Input: part model. Units: mm. Frame: model coordinates. A direction names the side the tool comes from. Give positions to 0.01 mm unless a question says otherwise; leave off trailing zeros. Write each loop counter-clockwise with the first axis right and the second up, starting at its lowest first coordinate (ties: lowest second). Pieces come first, ordered by that corner, then holes. Notation, with made-up numbers: (-7, 47.25) - (47, 47.25) arc R15 cw to (47, 72.25) - close; hole circle Ø8 at (78.25, 25.25). An arc over 180 degrees is marked (long way). Answer as a JSON object with one key per item and string values. Group by question number.
from build123d import *

# Parameters (mm, degrees)
SKETCH1_W           = 75
SKETCH1_H           = 80
BOSS_EXTRUDE1_DEPTH = 3
SKETCH2_W           = 17
SKETCH2_H           = 80
BOSS_EXTRUDE2_DEPTH = 3
SKETCH7_W           = 25
SKETCH7_H           = 80
SKETCH7_W_2         = 14.8
SKETCH7_H_2         = 17
BOSS_EXTRUDE6_DEPTH = 3
SKETCH8_W           = 21.55
SKETCH8_H           = 23.85
SKETCH8_W_2         = 17.55
SKETCH8_H_2         = 19.85
BOSS_EXTRUDE7_DEPTH = 10
SKETCH9_W           = 12.5
SKETCH9_H           = 2.5
CUT_EXTRUDE3_DEPTH  = 23.85
SKETCH10_W          = 1.375
SKETCH10_H          = 19.85
BOSS_EXTRUDE8_DEPTH = 6.5
SKETCH11_W          = 20
SKETCH11_H          = 80
SKETCH11_R          = 2.7
BOSS_EXTRUDE9_DEPTH = 3
SKETCH3_W           = 8
SKETCH3_H           = 15
BOSS_EXTRUDE3_DEPTH = 3
SKETCH5_W           = 69
SKETCH5_H           = 17
SKETCH5_R           = 2.6
SKETCH5_W_2         = 25
BOSS_EXTRUDE4_DEPTH = 3
SKETCH21_R          = 2.7
CUT_EXTRUDE5_DEPTH  = 3


with BuildPart() as part:
    # Sketch1 → Boss-Extrude1 (new body)
    with BuildSketch(Plane.XY):
        with Locations((0, 40)):
            Rectangle(SKETCH1_W, SKETCH1_H)
        Polygon((4.25, 23.5), (20.75, 23.5), (26.5, 30), (26.5, 72), (-1.5, 72), (-1.5, 30), align=None, mode=Mode.SUBTRACT)
    extrude(amount=BOSS_EXTRUDE1_DEPTH)

    # Sketch2 → Boss-Extrude2 (add)
    with BuildSketch(Plane(origin=(37.5, 0, 0), x_dir=(0, 0, -1), z_dir=(1, 0, 0))):
        with Locations((8.5, 40)):
            Rectangle(SKETCH2_W, SKETCH2_H)
    boss_extrude2 = extrude(amount=-BOSS_EXTRUDE2_DEPTH)

    # Mirror1: Boss-Extrude2 across plane
    add(boss_extrude2.mirror(Plane(origin=(0, 0, 0), x_dir=(0, 0, 1), z_dir=(1, 0, 0))))

    # Sketch7 → Boss-Extrude6 (add)
    with BuildSketch(Plane.XY.offset(3)):
        with Locations((50, 40)):
            Rectangle(SKETCH7_W, SKETCH7_H)
        with Locations((50, 48.001193432)):
            Rectangle(SKETCH7_W_2, SKETCH7_H_2, mode=Mode.SUBTRACT)
    extrude(amount=-BOSS_EXTRUDE6_DEPTH)

    # Sketch8 → Boss-Extrude7 (add)
    with BuildSketch(Plane(origin=(0, 0, 0), x_dir=(-1, 0, 0), z_dir=(0, 0, -1))):
        with Locations((-50, 48.001193432)):
            Rectangle(SKETCH8_W, SKETCH8_H)
        with Locations((-50, 48.001193432)):
            Rectangle(SKETCH8_W_2, SKETCH8_H_2, mode=Mode.SUBTRACT)
    extrude(amount=BOSS_EXTRUDE7_DEPTH)

    # Sketch9 → Cut-Extrude3 (cut)
    with BuildSketch(Plane(origin=(0, 59.926193432, 0), x_dir=(1, 0, 0), z_dir=(0, 1, 0))):
        with Locations((50, 4.75)):
            Rectangle(SKETCH9_W, SKETCH9_H)
    extrude(amount=-CUT_EXTRUDE3_DEPTH, mode=Mode.SUBTRACT)

    # Sketch10 → Boss-Extrude8 (add)
    with BuildSketch(Plane(origin=(0, 0, 0), x_dir=(-1, 0, 0), z_dir=(0, 0, -1))):
        with Locations((-41.9125, 48.001193432)):
            Rectangle(SKETCH10_W, SKETCH10_H)
        with Locations((-58.0875, 48.001193432)):
            Rectangle(SKETCH10_W, SKETCH10_H)
    extrude(amount=BOSS_EXTRUDE8_DEPTH)

    # Sketch11 → Boss-Extrude9 (add)
    with BuildSketch(Plane(origin=(62.5, 0, 0), x_dir=(0, 0, -1), z_dir=(1, 0, 0))):
        with Locations((7, 40)):
            Rectangle(SKETCH11_W, SKETCH11_H)
        with Locations((7, 15)):
            Circle(SKETCH11_R, mode=Mode.SUBTRACT)
        with Locations((7, 65)):
            Circle(SKETCH11_R, mode=Mode.SUBTRACT)
    extrude(amount=BOSS_EXTRUDE9_DEPTH)

    # Sketch3 → Boss-Extrude3 (add)
    with BuildSketch(Plane(origin=(0, 0, 0), x_dir=(-1, 0, 0), z_dir=(0, 0, -1))):
        with Locations((-30.5, 49)):
            Rectangle(SKETCH3_W, SKETCH3_H)
        with Locations((5.5, 49)):
            Rectangle(SKETCH3_W, SKETCH3_H)
    extrude(amount=BOSS_EXTRUDE3_DEPTH)

    # Sketch5 → Boss-Extrude4 (add)
    with BuildSketch(Plane.XZ):
        with Locations((0, -8.5)):
            Rectangle(SKETCH5_W, SKETCH5_H)
        with Locations((-17.5, -7)):
            Circle(SKETCH5_R, mode=Mode.SUBTRACT)
        with Locations((50, -8.5)):
            Rectangle(SKETCH5_W_2, SKETCH5_H)
        with Locations((50.5, -7)):
            Circle(SKETCH5_R, mode=Mode.SUBTRACT)
    boss_extrude4 = extrude(amount=-BOSS_EXTRUDE4_DEPTH)

    # Mirror2: Boss-Extrude4 across plane
    add(boss_extrude4.mirror(Plane(origin=(0, 40, 0), x_dir=(0, 0, 1), z_dir=(0, -1, 0))))

    # Sketch21 → Cut-Extrude5 (cut)
    with BuildSketch(Plane(origin=(-34.5, 0, 0), x_dir=(0, 0, -1), z_dir=(1, 0, 0))):
        with Locations((7, 15)):
            Circle(SKETCH21_R)
        with Locations((7, 65)):
            Circle(SKETCH21_R)
    extrude(amount=-CUT_EXTRUDE5_DEPTH, mode=Mode.SUBTRACT)


solid = part.part
1) Cut plane C-C on y = 51. Count the separate pieces of the cut face and the enclosed holes in it, and give its area (3 significant figures).
2) Cut plane B-B on x = 45.5. Return the cut outline in (y, z).
3) Line query: line 1 along X through (y, z) = (21, -7.25); line 2 along X through (y, z) = (44.5, -2.25) (3 decimals); line 3 along Y through (x, z) = (29, -2.25). Output: solid intervals per line, ascending. Write a range as from..to.
4) Mould query, pull axis X, two halves, no side actions, for faces 1 (the face through (43.75, 37, -5)), 2 (the face through (13, 0, -7)), 3 (the face through (-37.5, 41, -7)). Classes: +X half, -X half, draft (parallel to the pull), parting line (faces both ways), or undercut.
5) Reachability of faces 4 (the face through (-15.02, 1.48, -6.22)), 5 (the face through (63.979, 17.677, -6.649)), 6 (the face through (50, 59, -3.5)), 7 (the face through (50, 36.076, -7)) from +Z, -Z, +X, -X, +Y, -Y: full face, straight path, thin tool, end or side. Return the list, or none.
6) Cut plane A-A on y = 65. Return the cut outline in (x, z).
7) Pin query (flat end, axial travel): P1, Ø1.5, axis at x = 32.5, z = -1, coming from the -Y side; P2, Ø4, axis at x = 32, y = 49, coming from the -Z side; P3, Ø1.5, axis at x = 41.5, y = 43.5, coming from the -Z side; P4, Ø3, axis at y = 65, z = -7, coming from the +X side. Return the tip coordinate at first contact, or that it passes through.
8) Cut plane D-D on z = -13.25. Return the cut outline in (x, y).
Filled in:
{
 "1": {"separate pieces": "3", "enclosed holes": "0", "area": "439 mm²"},
 "2": {"outline": "(0, -17) - (3, -17) - (3, 0) - (36.08, 0) - (36.08, -3.5) - (38.08, -3.5) - (38.08, 0) - (39.5, 0) - (39.5, 3) - (0, 3) - close; (36.08, -10) - (38.08, -10) - (38.08, -6) - (36.08, -6) - close; (56.5, 0) - (57.93, 0) - (57.93, -3.5) - (59.93, -3.5) - (59.93, 0) - (77, 0) - (77, -17) - (80, -17) - (80, 3) - (56.5, 3) - close; (57.93, -10) - (59.93, -10) - (59.93, -6) - (57.93, -6) - close"},
 "3": {"line 1": "x = -37.5..-34.5, 34.5..37.5, 62.5..65.5", "line 2": "x = -37.5..-34.5, -9.5..-1.5, 26.5..37.5, 39.225..42.6, 57.4..60.775, 62.5..65.5", "line 3": "y = 0..3, 41.5..56.5, 77..80"},
 "4": {"face 1": "undercut", "face 2": "draft", "face 3": "-X half"},
 "5": {"face 4": "+Y, -Y", "face 5": "+X", "face 6": "none", "face 7": "-Z"},
 "6": {"outline": "(-37.5, -17) - (-34.5, -17) - (-34.5, -9.7) - (-37.5, -9.7) - close; (-37.5, -4.3) - (-34.5, -4.3) - (-34.5, 0) - (-1.5, 0) - (-1.5, 3) - (-37.5, 3) - close; (26.5, 0) - (34.5, 0) - (34.5, -17) - (37.5, -17) - (37.5, 0) - (62.5, 0) - (62.5, -4.3) - (65.5, -4.3) - (65.5, 3) - (26.5, 3) - close; (62.5, -17) - (65.5, -17) - (65.5, -9.7) - (62.5, -9.7) - close"},
 "7": {"P1": "stops at y = 0", "P2": "stops at z = -3", "P3": "stops at z = -10", "P4": "stops at x = 37.5"},
 "8": {"outline": "(-37.5, 0) - (65.5, 0) - (65.5, 80) - (-37.5, 80) - close; hole (-34.5, 3) - (34.5, 3) - (34.5, 77) - (-34.5, 77) - close; hole (37.5, 3) - (62.5, 3) - (62.5, 77) - (37.5, 77) - close"}
}
